Work out the finished part from the listing and answer in its coordinate system (mm). A direction names the side the tool comes from. Give positions to 0.01 mm unless a question says otherwise; leave off trailing zeros. Order: outer loops, then holes, each group sorted by start corner. A loop starts at its lowest first (then second) coordinate and runs counter-clockwise, first axis right, second up. Notation, with made-up numbers: (35, 66) -> (53, 66) arc R23 ccw to (53, 83) -> close; hole circle Ø9 at (-19.5, 62). An arc over 180 degrees is marked (long way). Answer as CSV lines item,"result". Start each with the question number.
1. A cutting plane is placed at D-D (z = -15.5). Give the vertices of the cut face in (x, y), then the cut area to 3 significant figures.
2. Find the intervals of material crossed by L1, parallel to X at y = 9.25, z = 0; L2, parallel to Z at x = 2, y = 5.5; L3, parallel to X at y = 6.75, z = 0, in increasing order.
3. For faces 4 (the cylindrical face through (10.74, 13.07, 2.38)), 5 (the flat face through (5, 5, 10)), 6 (the flat face through (0, 0, 3)), determine the directions among +Z, -Z, +X, -X, +Y, -Y from which every point of the face is accessible in a straight line to the end or side of a thin tool.
4. A cutting plane is placed at A-A (z = 0). Give the vertices of the cut face in (x, y).
5. A cutting plane is placed at B-B (x = -16). Give the vertices of the cut face in (y, z).
6. Flat-ended cylindrical pins translate along their axes: pin 1 (8.5 mm diameter, centred on x = 15.11, z = 8.72, fed in from +Y); pin 2 (6 mm diameter, centred on x = -4.5, y = 17, fed in from -Z); pin 3 (10 mm diameter, centred on x = 14, y = 13.5, fed in from -Z); pin 4 (3 mm diameter, centred on x = 0, z = 0, fed in from -Y). Find the tip coordinate at first contact, or state that the pin passes through.
7. A cutting plane is placed at C-C (y = 6.75). Give the vertices of the cut face in (x, z) (3 decimals).
8. For a pull along X with two mould halves and no side action, classify faces 1 (the flat face through (-3, 19, 0)), 2 (the cylindrical face through (10.74, 2.46, 2.38)), 3 (the cylindrical face through (2.44, 9.63, 0.54)) as released by +X, released by -X, zero draft, split by the parting line, or undercut.
from build123d import *

# Parameters (mm, degrees)
SKETCH2_R          = 2.65
CUT_EXTRUDE1_DEPTH = 34.571044071


with BuildPart() as part:
    # Sketch1 → Revolve1 (revolve)
    with BuildSketch(Plane.XY, mode=Mode.PRIVATE) as revolve1_sk:
        Polygon((-2.5, 0), (-2.5, 19), (-11, 19), (-11, 7.3), (-22.25, 7.3), (-22.25, 5), (-11, 5), (-11, 0), align=None)
    revolve(revolve1_sk.sketch.rotate(Axis((0, 0, 0), (0, 1, 0)), 270), axis=Axis((0, 0, 0), (0, 1, 0)))

    # Sketch2 → Cut-Extrude1 (cut, through all)
    with BuildSketch(Plane(origin=(0, 7.3, 0), x_dir=(1, 0, 0), z_dir=(0, 1, 0))):
        with Locations(Location((0, 17.45, 0), (0, 0, 270))):
            Circle(SKETCH2_R)
        with Locations(Location((15.112143296, -8.725, 0), (0, 0, 270))):
            Circle(SKETCH2_R)
        with Locations(Location((-15.112143296, -8.725, 0), (0, 0, 270))):
            Circle(SKETCH2_R)
    extrude(amount=-CUT_EXTRUDE1_DEPTH, mode=Mode.SUBTRACT)


solid = part.part
Answer sheet:
1,outline,"(-15.96, 5) -> (-1.79, 5) -> (-1.79, 7.3) -> (-15.96, 7.3) -> close; (1.79, 5) -> (15.96, 5) -> (15.96, 7.3) -> (1.79, 7.3) -> close"
1,area,"65.2 mm^2"
2,L1,"x = -11 to -2.5, 2.5 to 11"
2,L2,"z = -22.16 to -19.19, -15.71 to -1.5, 1.5 to 22.16"
2,L3,"x = -22.25 to -2.5, 2.5 to 22.25"
3,face 4,"+Y"
3,face 5,"-Y"
3,face 6,"+Z, -Z, +X, -X, -Y"
4,outline,"(-22.25, 5) -> (-11, 5) -> (-11, 0) -> (-2.5, 0) -> (-2.5, 19) -> (-11, 19) -> (-11, 7.3) -> (-22.25, 7.3) -> close; (2.5, 0) -> (11, 0) -> (11, 5) -> (22.25, 5) -> (22.25, 7.3) -> (11, 7.3) -> (11, 19) -> (2.5, 19) -> close"
5,outline,"(5, -15.46) -> (7.3, -15.46) -> (7.3, 6.23) -> (5, 6.23) -> close; (5, 11.22) -> (7.3, 11.22) -> (7.3, 15.46) -> (5, 15.46) -> close"
6,pin 1,"stops at y = 7.3"
6,pin 2,"stops at z = -10.9"
6,pin 3,"stops at z = -6.32"
6,pin 4,"passes through"
7,outline,"circle Ø44.5 at (0, 0); hole circle Ø5.3 at (-15.112, 8.725); hole circle Ø5.3 at (0, -17.45); hole circle Ø5 at (0, 0); hole circle Ø5.3 at (15.112, 8.725)"
8,face 1,"zero draft"
8,face 2,"split by the parting line"
8,face 3,"undercut"
